from build123d import *

# Parameters (mm, degrees)
BOSS_EXTRU_1_DEPTH      = 3
BOSS_EXTRU_2_DEPTH      = 1.5
ESQUISSE3_W             = 15
ESQUISSE3_H             = 15
BOSS_EXTRU_3_DEPTH      = 10
ESQUISSE4_R             = 2
ENL_V_MAT_EXTRU_1_DEPTH = 10
ENL_V_MAT_EXTRU_2_DEPTH = 3


with BuildPart() as part:
    # Esquisse1 → Boss.-Extru.1 (new body)
    with BuildSketch(Plane.XY):
        Polygon((26.306445504, -26.841854987), (-41.693554496, -26.841854987), (-41.693554496, 7.023864035), (-57.693554496, 7.023864035), (-57.693554496, -34.841854987), (-41.693554496, -34.841854987), (26.306445504, -34.841854987), (36.306445504, -34.841854987), (36.306445504, 10.158145013), (26.306445504, 10.158145013), align=None)
    extrude(amount=BOSS_EXTRU_1_DEPTH)

    # Esquisse2 → Boss.-Extru.2 (add)
    with BuildSketch(Plane.XY.offset(3)):
        Polygon((-57.693554496, 7.023864035), (-57.693554496, -34.841854987), (36.306445504, -34.841854987), (36.306445504, 10.158145013), (30.306445504, 10.158145013), (30.306445504, -28.841854987), (-51.693554496, -28.841854987), (-51.693554496, 7.023864035), align=None)
    extrude(amount=BOSS_EXTRU_2_DEPTH)

    # Symétrie3: part across plane


with BuildPart() as part_1:
    add(part.part)
    add(part.part.mirror(Plane.XY.offset(4.5)))

    # Esquisse3 → Boss.-Extru.3 (add)
    with BuildSketch(Plane.XZ.offset(34.841854987)):
        with Locations((-50.193554496, 16.5)):
            Rectangle(ESQUISSE3_W, ESQUISSE3_H)
        with Locations((28.806445504, 16.5)):
            Rectangle(ESQUISSE3_W, ESQUISSE3_H)
    extrude(amount=-BOSS_EXTRU_3_DEPTH)

    # Esquisse4 → Enlèv. mat.-Extru.1 (cut)
    with BuildSketch(Plane(origin=(0, -24.841854987, 0), x_dir=(1, 0, 0), z_dir=(0, 1, 0))):
        with Locations((-50.193554496, -16.5)):
            Circle(ESQUISSE4_R)
        with Locations((28.806445504, -16.5)):
            Circle(ESQUISSE4_R)
    extrude(amount=-ENL_V_MAT_EXTRU_1_DEPTH, mode=Mode.SUBTRACT)

    # Esquisse5 → Enlèv. mat.-Extru.2 (cut)
    with BuildSketch(Plane(origin=(0, -24.841854987, 0), x_dir=(1, 0, 0), z_dir=(0, 1, 0))):
        Polygon((-51.839002763, -13.65), (-48.548106229, -13.65), (-46.902657962, -16.5), (-48.548106229, -19.35), (-51.839002763, -19.35), (-53.484451031, -16.5), align=None)
        Polygon((27.160997237, -13.65), (30.451893771, -13.65), (32.097342038, -16.5), (30.451893771, -19.35), (27.160997237, -19.35), (25.515548969, -16.5), align=None)
    extrude(amount=-ENL_V_MAT_EXTRU_2_DEPTH, mode=Mode.SUBTRACT)


solid = part_1.part
Input: part model. Units: mm. Frame: model coordinates. A direction names the side the tool comes from. Coordinates: 2 decimals unless noted, no trailing zeros. Loops run counter-clockwise (first coordinate to the right, second up) from the corner with the lowest first, then second, coordinate; pieces in that order, holes last.
Q1. Contact query for flat-ended pins moving along their axis: pin 1 (0.9 mm diameter, centred on x = -21, z = 7.5, fed in from +Y); pin 2 (2 mm diameter, centred on x = -12.5, y = -25.5, fed in from +Z); pin 3 (5 mm diameter, centred on x = 24.5, z = 13.5, fed in from +Y); pin 4 (12 mm diameter, centred on x = -51.5, z = 13.5, fed in from +Y). Output: stop coordinate, or through.
Q2. Draft query along Z for faces 6 (the face through (-41.694, -10, 8)), 7 (the face through (-47.737, -26.321, 15.055)), 8 (the face through (24, -26, 9)). Return one class per face: +Z half, -Z half, draft (parallel to the pull), parting line (faces both ways), or undercut.
Q3. Cut plane D-D (z = 15.5). Output: boundary loops of the cut face in (x, y), then the cut area to 3 significant figures.
Q4. Cut plane A-A (z = 11). Output: boundary loops of the cut face in (x, y), then the cut area to 3 significant figures.
Q5. Set-up query: faces 1 (the face through (-51.694, -11, 5)), 2 (the face through (-11, -27, 0)), 3 (the face through (27.33, -31.29, 15.15)), 4 (the face through (21.306, -30, 16)), 5 (the face through (-49.6, 7.024, 2.6)). Return all of +Z, -Z, +X, -X, +Y, -Y with unobstructed straight access to the full face (end or side cutting, diameter ignored); none if empty.
Q6. Material intervals for line 1 (X direction, y = -32.5, z = 16.5); line 2 (X direction, y = -20, z = 2.5); line 3 (X direction, y = -27, z = 22.5), sorted ascending.
Q7. Cut plane C-C (x = -8). Output: boundary loops of the cut face in (y, z), then the cut area to 3 significant figures.
Q8. Cut plane B-B (y = 4). Output: boundary loops of the cut face in (x, z), then the cut area to 3 significant figures.
Working result:
1. pin 1: stops at y = -26.84
1. pin 2: passes through
1. pin 3: stops at y = -24.84
1. pin 4: stops at y = 7.02
2. face 6: draft
2. face 7: undercut
2. face 8: -Z half
3. outline: (-57.69, -34.84) - (-51.93, -34.84) - (-51.93, -27.84) - (-52.91, -27.84) - (-52.91, -24.84) - (-57.69, -24.84) - close; (-48.46, -34.84) - (-42.69, -34.84) - (-42.69, -24.84) - (-47.48, -24.84) - (-47.48, -27.84) - (-48.46, -27.84) - close; (21.31, -34.84) - (27.07, -34.84) - (27.07, -27.84) - (26.09, -27.84) - (26.09, -24.84) - (21.31, -24.84) - close; (30.54, -34.84) - (36.31, -34.84) - (36.31, -24.84) - (31.52, -24.84) - (31.52, -27.84) - (30.54, -27.84) - close
3. area: 219 mm2
4. outline: (-57.69, -34.84) - (-42.69, -34.84) - (-42.69, -24.84) - (-57.69, -24.84) - close; (21.31, -34.84) - (36.31, -34.84) - (36.31, -24.84) - (21.31, -24.84) - close
4. area: 300 mm2
5. face 1: +Y
5. face 2: -Z, +X, -X, +Y, -Y
5. face 3: +Y, -Y
5. face 4: +Z, +Y, -Y
5. face 5: +Z, -Z, -X, +Y
6. line 1: x = -57.69 to -52.19, -48.19 to -42.69, 21.31 to 26.81, 30.81 to 36.31
6. line 2: x = -57.69 to -41.69, 26.31 to 36.31
6. line 3: x = -57.69 to -42.69, 21.31 to 36.31
7. outline: (-34.84, 0) - (-26.84, 0) - (-26.84, 3) - (-28.84, 3) - (-28.84, 6) - (-26.84, 6) - (-26.84, 9) - (-34.84, 9) - close
7. area: 66.0 mm2
8. outline: (-57.69, 0) - (-41.69, 0) - (-41.69, 3) - (-51.69, 3) - (-51.69, 6) - (-41.69, 6) - (-41.69, 9) - (-57.69, 9) - close; (26.31, 0) - (36.31, 0) - (36.31, 9) - (26.31, 9) - (26.31, 6) - (30.31, 6) - (30.31, 3) - (26.31, 3) - close
8. area: 192 mm2
